from build123d import *

# Parameters (mm, degrees)
F0_R     = 30
F0_R_2   = 20
F1_DEPTH = 45
F2_R     = 4.99999


# Not quite as in the source:
# - a fillet or chamfer is up to 0.001 mm smaller than in the source, because OpenCascade refuses the exact size


with BuildPart() as f1:
    # F0 (on Top) → F1 (new body)
    with BuildSketch(Plane.XY):
        with Locations((0, -1.9317325205)):
            Circle(F0_R)
        with Locations((0, -1.9317325205)):
            Circle(F0_R_2, mode=Mode.SUBTRACT)
    extrude(amount=F1_DEPTH)

    # F2 (radius 5 in the source; OpenCascade refuses exactly that, so slightly less here)
    f2_edges = [f1.edges().sort_by_distance(p)[0] for p in [
        (-30, -1.931733, 0),
        (-20, -1.931733, 0),
        (-20, -1.931733, 45),
        (-30, -1.931733, 45),
    ]]
    fillet(f2_edges, radius=F2_R)


solid = f1.part
CAD build for the part. Positions are in the model's coordinates, mm. Give positions to 0.01 mm unless a question says otherwise; leave off trailing zeros. Write each loop counter-clockwise with the first axis right and the second up, starting at its lowest first coordinate (ties: lowest second). Pieces come first, ordered by that corner, then holes. Notation, with made-up numbers: (60.25, 50) - (119.25, 50) arc R19 ccw to (119.25, 67) - close; hole circle Ø7 at (2, 18.5). An arc over 180 degrees is marked (long way). Put each result on its own line as item: value.
(1) Saw through at B-B (z = 38.5). List the corners of the cut face in (x, y), then the cut area to 3 significant figures.
Working result:
outline: circle Ø60 at (0, -1.93); hole circle Ø40 at (0, -1.93)
area: 1,570 mm^2
(2) Wall check: L1, parallel to Y at x = 0, z = 19; L2, parallel to X at y = -2, z = 14; L3, parallel to Y at x = 7, z = 6.5. Give the ranges that are in metal, low to high.
Working result:
L1: -31.93 to -21.93, 18.07 to 28.07
L2: -30 to -20, 20 to 30
L3: -31.1 to -20.67, 16.8 to 27.24
(3) Pull direction X, two halves, no side cores. Call faces 1 (the cylindrical face through (-29.97, -0.61, 22.25)), 2 (the cylindrical face through (10.8, 14.9, 22.3)): released by +X, released by -X, zero draft, split by the parting line, or undercut.
Working result:
face 1: split by the parting line
face 2: undercut
(4) Drop flat-ended pins along their axis: pin 1 Ø3 at (y, z) = (9.5, 40.5) entering from +X; pin 2 Ø4 at (x, z) = (17, 23.5) entering from +Y; pin 3 Ø12 at (x, z) = (9, 8.5) entering from -Y; pin 4 Ø12 at (y, z) = (-5, 37) entering from -X. Give the stop position or say it passes through.
Working result:
pin 1: x = 28.29
pin 2: y = 24.05
pin 3: y = -31.78
pin 4: x = -30
